```python
from build123d import *

# Parameters (mm, degrees)
SKETCH1_W                  = 28.76
SKETCH1_H                  = 34.79
PCB_DEPTH                  = 1.56
F_3_8_3_8_DIAMETER_HOLE4_D = 3.8
SKETCH7_W                  = 2.38
SKETCH7_H                  = 20.5
HEADERS_DEPTH              = 4.43
SKETCH8_R                  = 0.5
CUT_EXTRUDE1_DEPTH         = 23.999898369
FILLET1_R                  = 2


with BuildPart() as part:
    # Sketch1 → PCB (new body)
    with BuildSketch(Plane(origin=(0, 0, 0), x_dir=(1, 0, 0), z_dir=(0, 1, 0))):
        Rectangle(SKETCH1_W, SKETCH1_H)
    extrude(amount=PCB_DEPTH)

    # Ø3.8 (3.8) Diameter Hole4 (through all)
    with Locations(Plane(origin=(0, 1.56, 0), x_dir=(1, 0, 0), z_dir=(0, 1, 0))):
        with Locations((-11.375, 12.955), (11.375, 12.955), (-11.375, -14.975), (11.375, -14.975)):
            Hole(F_3_8_3_8_DIAMETER_HOLE4_D / 2)

    # Sketch7 → Headers (add)
    with BuildSketch(Plane(origin=(0, 1.56, 0), x_dir=(1, 0, 0), z_dir=(0, 1, 0))):
        with Locations((-11.203491178, -0.781399088)):
            Rectangle(SKETCH7_W, SKETCH7_H)
    headers = extrude(amount=HEADERS_DEPTH)

    # Sketch8 → Cut-Extrude1 (cut, through all)
    with BuildSketch(Plane(origin=(0, 1.56, 0), x_dir=(1, 0, 0), z_dir=(0, 1, 0))):
        with Locations(Location((-6.541275499, -16.295, 0), (0, 0, 270))):
            Circle(SKETCH8_R)
        with Locations(Location((-4.001275499, -16.295, 0), (0, 0, 270))):
            Circle(SKETCH8_R)
        with Locations(Location((-1.461275499, -16.295, 0), (0, 0, 270))):
            Circle(SKETCH8_R)
        with Locations(Location((1.078724501, -16.295, 0), (0, 0, 270))):
            Circle(SKETCH8_R)
        with Locations(Location((3.618724501, -16.295, 0), (0, 0, 270))):
            Circle(SKETCH8_R)
        with Locations(Location((6.158724501, -16.295, 0), (0, 0, 270))):
            Circle(SKETCH8_R)
    extrude(amount=-CUT_EXTRUDE1_DEPTH, mode=Mode.SUBTRACT)

    # Mirror1: Headers across plane
    add(headers.mirror(Plane(origin=(0, 0, 0), x_dir=(0, 0, 1), z_dir=(1, 0, 0))))

    # Fillet1
    fillet1_edges = [part.edges().sort_by_distance(p)[0] for p in [
        (14.38, 0.78, 17.395),
        (-14.38, 0.78, 17.395),
        (-14.38, 0.78, -17.395),
        (14.38, 0.78, -17.395),
    ]]
    fillet(fillet1_edges, radius=FILLET1_R)


solid = part.part
```
The listing builds one solid part. Answer for the finished solid, in the listing's coordinates (mm). A direction names the side the tool comes from. Give positions to 0.01 mm unless a question says otherwise; leave off trailing zeros. Loops run counter-clockwise (first coordinate to the right, second up) from the corner with the lowest first, then second, coordinate; pieces in that order, holes last. Notation, with made-up numbers: (-8, 24.5) - (11, 24.5) arc R16 cw to (11, 41.5) - close; hole circle Ø2 at (-8.5, 59). An arc over 180 degrees is marked (long way). Return JSON: item names as keys, results as strings. Group by question number.
1. Given pin 1 Ø1.9 at (x, y) = (-11, 4) entering from -Z; pin 2 Ø3.5 at (y, z) = (3.5, 3) entering from -X; pin 3 Ø3 at (x, z) = (11.375, 14.975) entering from +Y; pin 4 Ø0.7 at (x, y) = (11.5, 3) entering from +Z, each flat-ended and moving along its own axis, determine where each tip first touches the part or whether it passes through.
2. Find section A-A (y = 4.35). Write down the section's boundary in (x, z).
3. Find section D-D (z = -12.5). Write down the section's boundary in (x, y).
4. Determine the mould class of faces 4 (the flat face through (-11, 4, 11.031)), 5 (the flat face through (12.393, 4, 1)), 6 (the cylindrical face through (-6.519, 0.791, 15.795)) for opening direction Z: pulls with the +Z half, pulls with the -Z half, needs draft (parallel to the pull), parting line crosses it, or undercut.
5. Which of the six approach directions +Z, -Z, +X, -X, +Y, -Y give full straight-line access (tool end or side, diameter ignored) to faces 1 (the flat face through (10.013, 4, 1)), 2 (the cylindrical face through (-1.4, 0.8, 15.8)), 3 (the flat face through (-12.393, 4, 1))?
6. Find section B-B (x = -10.5). Write down the section's boundary in (y, z) (3 decimals), then the cut area to 3 significant figures.
7. Find section C-C (z = 8). Write down the section's boundary in (x, y), then the cut area to 3 significant figures.
8. Straight lines are drawn through the part: line 1 (Z direction, x = 11.25, y = 1.1) (3 decimals); line 2 (X direction, y = 5.4, z = 10); line 3 (Z direction, x = 10.75, y = 3.3). For each, find the intervals that lie inside material, in ascending order. Write a range as [from, to].
Verdict:
{
 "1": {"pin 1": "stops at z = -9.47", "pin 2": "stops at x = -12.39", "pin 3": "passes through", "pin 4": "stops at z = 11.03"},
 "2": {"outline": "(-12.39, -9.47) - (-10.01, -9.47) - (-10.01, 11.03) - (-12.39, 11.03) - close; (10.01, -9.47) - (12.39, -9.47) - (12.39, 11.03) - (10.01, 11.03) - close"},
 "3": {"outline": "(-14.38, 0) - (-13.22, 0) - (-13.22, 1.56) - (-14.38, 1.56) - close; (-9.53, 0) - (9.53, 0) - (9.53, 1.56) - (-9.53, 1.56) - close; (13.22, 0) - (14.38, 0) - (14.38, 1.56) - (13.22, 1.56) - close"},
 "4": {"face 4": "pulls with the +Z half", "face 5": "needs draft", "face 6": "undercut"},
 "5": {"face 1": "+Z, -Z, +Y", "face 2": "+Y, -Y", "face 3": "+Z, -Z, -X, +Y"},
 "6": {"outline": "(0, -17.395) - (1.56, -17.395) - (1.56, -14.642) - (0, -14.642) - close; (0, -11.268) - (1.56, -11.268) - (1.56, -9.469) - (5.99, -9.469) - (5.99, 11.031) - (1.56, 11.031) - (1.56, 13.288) - (0, 13.288) - close; (0, 16.662) - (1.56, 16.662) - (1.56, 17.395) - (0, 17.395) - close", "area": "135 mm^2"},
 "7": {"outline": "(-14.38, 0) - (14.38, 0) - (14.38, 1.56) - (12.39, 1.56) - (12.39, 5.99) - (10.01, 5.99) - (10.01, 1.56) - (-10.01, 1.56) - (-10.01, 5.99) - (-12.39, 5.99) - (-12.39, 1.56) - (-14.38, 1.56) - close", "area": "66.0 mm^2"},
 "8": {"line 1": "z = [-17.395, -14.851], [-11.059, 13.079], [16.871, 17.395]", "line 2": "x = [-12.39, -10.01], [10.01, 12.39]", "line 3": "z = [-9.47, 11.03]"}
}
